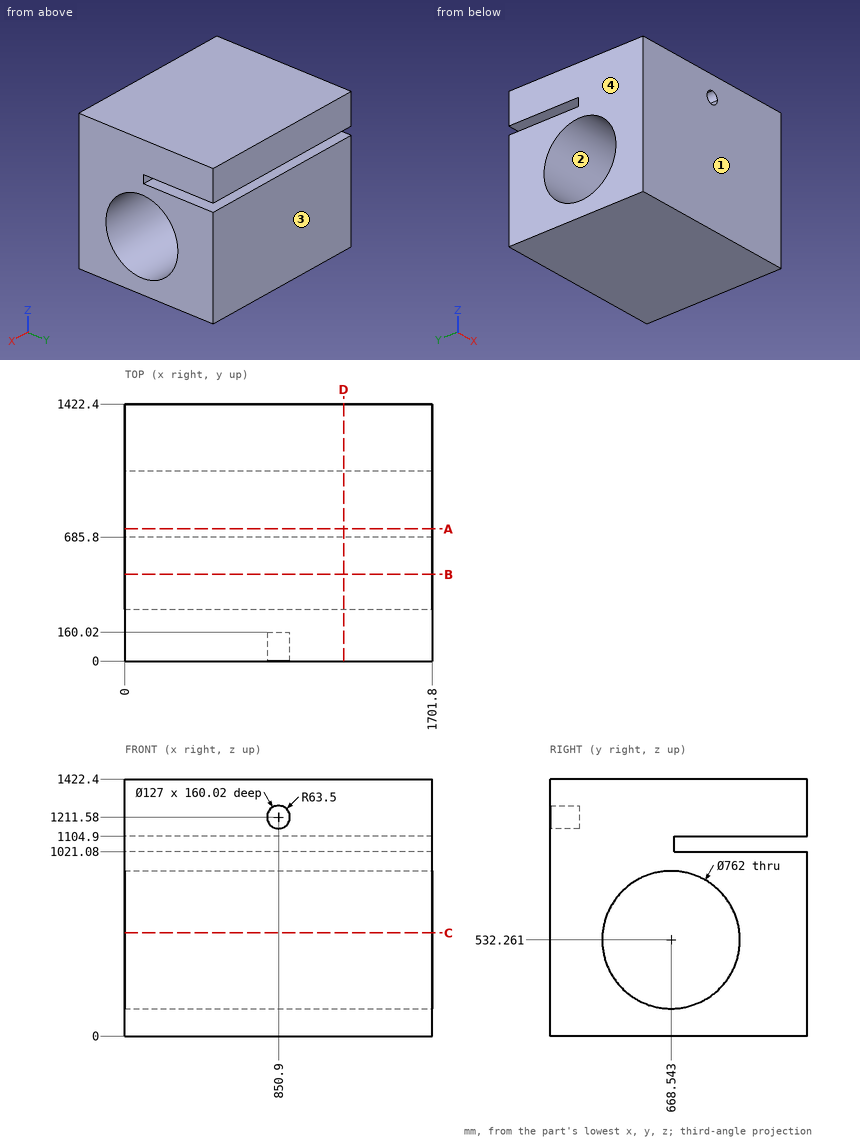
Verification items for this drawing (mm, ordinates from the low corner). Give positions to 0.01 mm unless a question says otherwise; leave off trailing zeros. Loops run counter-clockwise (first coordinate to the right, second up) from the corner with the lowest first, then second, coordinate; pieces in that order, holes last. Notation, with made-up numbers: M 20.25,-20.75 L 79.25,-20.75 A22 ccw 79.25,4.25 Z; hole C 86.25,41.25 d3. An arc over 180 degrees is marked long. Answer as a JSON object with one key per item and string values. Group by question number.
Item 1: Gauge pin test, flat ends, axial feed: pin 1 (25 mm diameter, centred on x = 546, z = 1061, fed in from +Y); pin 2 (12 mm diameter, centred on x = 1515, y = 871.5, fed in from -Z). Record the tip position at first contact, or that the pin passes through.
Item 2: Sectioned sample at B-B on y = 479. Record the boundary of the cut face in (x, z) (1 decimal).
Item 3: Material ranges on L1, parallel to X at y = 91.5, z = 1211.58; L2, parallel to Z at x = 1132, y = 1158; L3, parallel to Z at x = 1136, y = 942.5, recorded low to high.
Item 4: Sectioned sample at D-D on x = 1212. Record the boundary of the cut face in (y, z), plus the area to 3 significant figures.
Item 5: Sectioned sample at C-C on z = 571. Record the boundary of the cut face in (x, y), plus the area to 3 significant figures.
Item 6: Mould release check, pull along Y, two halves, no side actions. Record for the marked faces 1, 2, 3 and 4: pulls with the +Y half, pulls with the -Y half, needs draft (parallel to the pull), parting line crosses it, or undercut.
Item 7: Sectioned sample at A-A on y = 731.5. Record the boundary of the cut face in (x, z), plus the area to 3 significant figures.
Findings below:
{
 "1": {"pin 1": "y = 685.8", "pin 2": "z = 0"},
 "2": {"outline": "M 0,0 L 1701.8,0 L 1701.8,201.8 L 0,201.8 Z; M 0,862.8 L 1701.8,862.8 L 1701.8,1422.4 L 0,1422.4 Z"},
 "3": {"L1": "0 to 787.4, 914.4 to 1701.8", "L2": "0 to 1021.08, 1104.9 to 1422.4", "L3": "0 to 267.48, 797.04 to 1021.08, 1104.9 to 1422.4"},
 "4": {"outline": "M 0,0 L 1422.4,0 L 1422.4,1021.08 L 685.8,1021.08 L 685.8,1104.9 L 1422.4,1104.9 L 1422.4,1422.4 L 0,1422.4 Z; hole C 668.54,532.26 d762", "area": "1,510,000 mm2"},
 "5": {"outline": "M 0,0 L 1701.8,0 L 1701.8,289.52 L 0,289.52 Z; M 0,1047.57 L 1701.8,1047.57 L 1701.8,1422.4 L 0,1422.4 Z", "area": "1,130,000 mm2"},
 "6": {"face 1": "pulls with the -Y half", "face 2": "undercut", "face 3": "pulls with the +Y half", "face 4": "needs draft"},
 "7": {"outline": "M 0,0 L 1701.8,0 L 1701.8,156.5 L 0,156.5 Z; M 0,908.02 L 1701.8,908.02 L 1701.8,1021.08 L 0,1021.08 Z; M 0,1104.9 L 1701.8,1104.9 L 1701.8,1422.4 L 0,1422.4 Z", "area": "999,000 mm2"}
}
